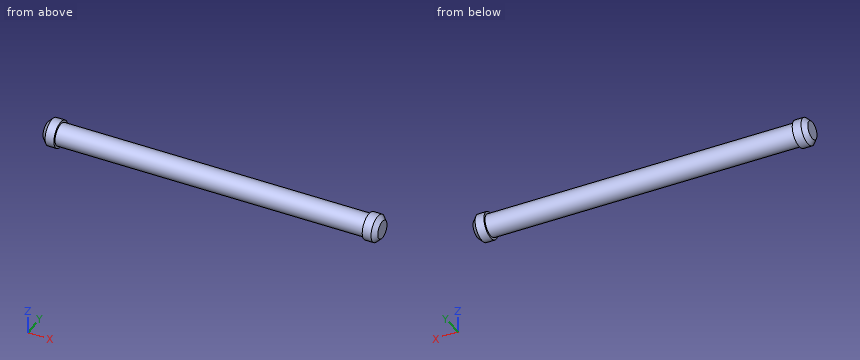
Autodesk Inventor part; units mm, degrees
ref_plane "YZ Plane" through (0, 0, 0) normal (1, 0, 0) x (0, 1, 0)
ref_plane "XZ Plane" through (0, 0, 0) normal (0, 1, 0) x (-1, 0, 0)
ref_plane "XY Plane" through (0, 0, 0) normal (0, 0, 1) x (1, 0, 0)
sketch "Sketch1" plane through (0, 0, 0) normal (1, 0, 0) x (0, 1, 0)
  circle A0 centre (0, 0) radius 3.175
  dimension "d0" = 6.35
extrude "Extrusion1" add sketch "Sketch1" along normal mid plane 88.9
sketch "Sketch2" plane through (44.45, 0, 0) normal (1, 0, 0) x (0, 0, -1)
  circle A0 centre (0, 0) radius 3.81
  dimension "d3" = 7.62
extrude "Extrusion2" add sketch "Sketch2" along normal blind 3.81
chamfer "Chamfer1" distance 1.27 angle 45 1 edges at (48.26, 0, 3.81)
mirror "Mirror1" about plane through (0, 0, 0) normal (1, 0, 0) of "Extrusion2", "Chamfer1"
properties part number "PivetRob(H)"
For this review, take the finished solid that the model builds, in its own axes (mm). Coordinates: 2 decimals unless noted, no trailing zeros. Write each loop counter-clockwise with the first axis right and the second up, starting at its lowest first coordinate (ties: lowest second). Pieces come first, ordered by that corner, then holes. Notation, with made-up numbers: (-37.5, 27.25) -> (6.5, 27.25) arc R20 ccw to (6.5, 61.25) -> close; hole circle Ø1 at (25, -4.75). An arc over 180 degrees is marked (long way). Put each result on its own line as item: value.
Q1. Wall thickness on L1, parallel to Y at x = 41.5, z = -0.25; L2, parallel to X at y = -0.5, z = 3.5: over which ranges is each line inside the solid? List them lowest first.
From the geometry:
L1: y = -3.17 to 3.17
L2: x = -47.26 to -44.45, 44.45 to 47.26
Q2. Take a section at A-A, the plane z = 0. State the section outline as (x, y) points (3 decimals).
From the geometry:
outline: (-48.26, -2.54) -> (-46.99, -3.81) -> (-44.45, -3.81) -> (-44.45, -3.175) -> (44.45, -3.175) -> (44.45, -3.81) -> (46.99, -3.81) -> (48.26, -2.54) -> (48.26, 2.54) -> (46.99, 3.81) -> (44.45, 3.81) -> (44.45, 3.175) -> (-44.45, 3.175) -> (-44.45, 3.81) -> (-46.99, 3.81) -> (-48.26, 2.54) -> close
Q3. Take a section at C-C, the plane x = 8.5. State the section outline as (y, z) points (3 decimals).
From the geometry:
outline: circle Ø6.35 at (0, 0)
Q4. Clearance check with flat-ended pins moving along their axes: pin 1 Ø4 at (x, y) = (-17.5, -1) entering from -Z (3 decimals); pin 2 Ø1.5 at (x, y) = (-28, -3) entering from +Z; pin 3 Ø1 at (y, z) = (2.5, 2) entering from +X. State where each tip first meets the part, or that it passes through.
From the geometry:
pin 1: stops at z = -3.175
pin 2: stops at z = 2.24
pin 3: stops at x = 48.1
